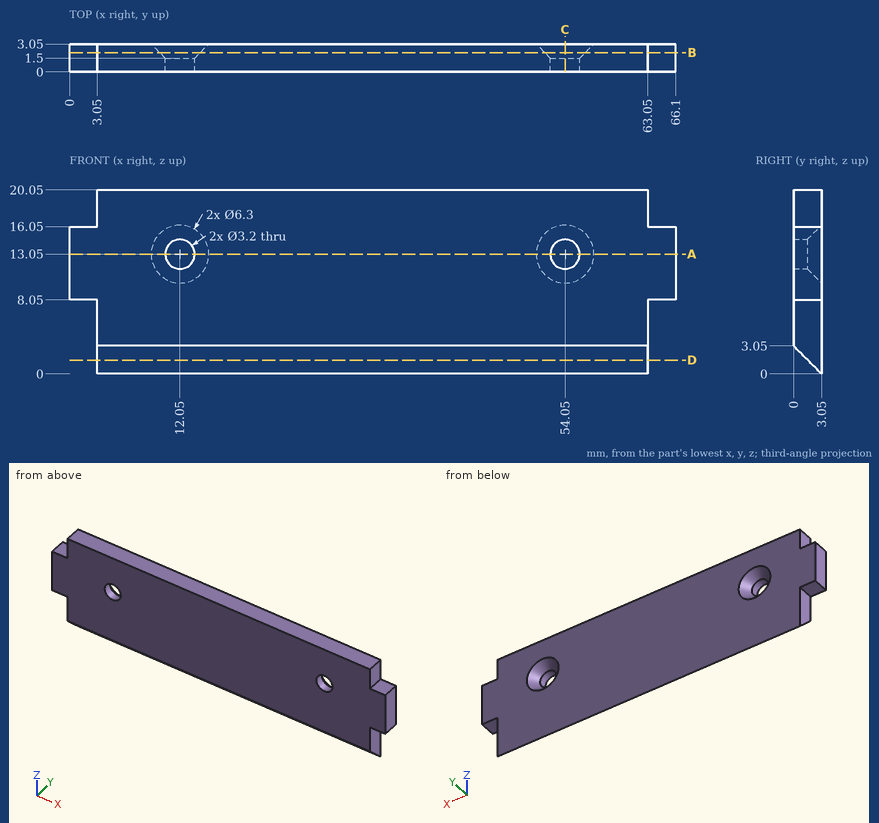
Can you work these out from the drawing? Everything is in mm from the part's minimum corner. Coordinates: 2 decimals unless noted, no trailing zeros. Loops run counter-clockwise (first coordinate to the right, second up) from the corner with the lowest first, then second, coordinate; pieces in that order, holes last. Notation, with made-up numbers: M 24,89.25 L 39,89.25 A21 ccw 39,118.25 Z; hole C 25.5,4 d9. An arc over 180 degrees is marked long. One line per item, written item: value.
1. Imagine slicing it at C-C (x = 54.05). List the corners of the cut face in (y, z) for me.
Geometry says:
outline: M 0,3.05 L 3.05,0 L 3.05,9.9 L 1.5,11.45 L 0,11.45 Z; M 0,14.65 L 1.5,14.65 L 3.05,16.2 L 3.05,20.05 L 0,20.05 Z
2. Will these pins go through, and if not, where does the flat tip stop? pin 1 Ø1 at (x, z) = (36, 16.5) entering from -Y; pin 2 Ø1.5 at (y, z) = (2.5, 5) entering from +X; pin 3 Ø5 at (x, z) = (12.05, 13.05) entering from +Y; pin 4 Ø0.9 at (x, y) = (2, 1.5) entering from -Z.
Geometry says:
pin 1: stops at y = 0
pin 2: stops at x = 63.05
pin 3: stops at y = 2.4
pin 4: stops at z = 8.05
3. Please list where these lines run through material, in increasing order: probe 1 along X at (y, z) = (0.5, 13.05); probe 2 along X at (y, z) = (0.8, 14); probe 3 along X at (y, z) = (1.55, 6.5).
Geometry says:
probe 1: x = 0 to 10.45, 13.65 to 52.45, 55.65 to 66.1
probe 2: x = 0 to 10.76, 13.34 to 52.76, 55.34 to 66.1
probe 3: x = 3.05 to 63.05
4. Imagine slicing it at D-D (z = 1.5). List the corners of the cut face in (x, y) for me, and give its area (3 significant figures).
Geometry says:
outline: M 3.05,1.55 L 63.05,1.55 L 63.05,3.05 L 3.05,3.05 Z
area: 90.0 mm2
5. Imagine slicing it at A-A (z = 13.05). List the corners of the cut face in (x, y) for me, and give its area (3 significant figures).
Geometry says:
outline: M 0,0 L 10.45,0 L 10.45,1.5 L 8.9,3.05 L 0,3.05 Z; M 13.65,0 L 52.45,0 L 52.45,1.5 L 50.9,3.05 L 15.2,3.05 L 13.65,1.5 Z; M 55.65,0 L 66.1,0 L 66.1,3.05 L 57.2,3.05 L 55.65,1.5 Z
area: 177 mm2
6. Imagine slicing it at B-B (y = 2.1). List the corners of the cut face in (x, z) for me.
Geometry says:
outline: M 0,8.05 L 3.05,8.05 L 3.05,0.95 L 63.05,0.95 L 63.05,8.05 L 66.1,8.05 L 66.1,16.05 L 63.05,16.05 L 63.05,20.05 L 3.05,20.05 L 3.05,16.05 L 0,16.05 Z; hole C 12.05,13.05 d4.4; hole C 54.05,13.05 d4.4
